CAD build for the part. Positions are in the model's coordinates, mm. A direction names the side the tool comes from. Give positions to 0.01 mm unless a question says otherwise; leave off trailing zeros. Loops run counter-clockwise (first coordinate to the right, second up) from the corner with the lowest first, then second, coordinate; pieces in that order, holes last. Notation, with made-up numbers: M -38.75,-17.75 L -17.75,-17.75 A35 cw -17.75,15.25 Z; hole C -26.5,54 d2. An arc over 180 degrees is marked long. Answer as CSV lines item,"result".
```python
from build123d import *

# Parameters (mm, degrees)
F2_R            = 1.27
F5_D            = 4.826
F5_DEPTH        = 7.62
F5_START        = 0.0546078
F5_TIP          = 1.4498766737
F5_COPIES_COUNT = 5


# Not quite as in the source:
# - a pattern or mirror of a feature is missing from the dataset's text; its kind, count and spacing are read off the source's solid


with BuildPart() as f1:
    # F0 (on Right) → F1 (revolve)
    with BuildSketch(Plane.YZ):
        Polygon((-6.35, 50.8), (6.35, 50.8), (6.35, 53.34), (-8.89, 53.34), (-8.89, 40.64), (-135.9245181084, 40.64), (-141.0045181084, 40.64), (-141.0045181084, 0), (-135.9245181084, 0), (-135.9245181084, 38.1), (-6.35, 38.1), align=None)
    revolve(axis=Axis((0, -59.97428298, 0), (0, -1, 0)))

    # F2
    f2_edges = [f1.edges().sort_by_distance(p)[0] for p in [
        (0, -6.35, -38.1),
        (0, -6.35, -50.8),
        (0, -8.89, -40.64),
        (0, -135.924518, -38.1),
    ]]
    fillet(f2_edges, radius=F2_R)

    # F5
    # its depths count from where the whole tool has entered the part; down to there all is cleared
    with Locations(Plane.XY.offset(53.34).offset(-F5_START)):
        with Locations((0, 0)):
            f5 = Hole(F5_D / 2, depth=F5_DEPTH)
            with Locations((0, 0, -(F5_DEPTH + F5_TIP / 2))):  # 118° drill point
                Cone(0, F5_D / 2, F5_TIP, mode=Mode.SUBTRACT)

    # F5_copies: F5 ×5 about axis
    f5_copies_axis = Axis((0, 0, 0), (0, 1, 0))
    for i in range(1, F5_COPIES_COUNT):
        add(f5.rotate(f5_copies_axis, i * 360 / F5_COPIES_COUNT), mode=Mode.SUBTRACT)


solid = f1.part
```
Q1. Pin check, flat tips, straight feed: P1, Ø5, axis at x = -32, y = -77.5, coming from the -Z side; P2, Ø4, axis at x = -9.5, y = -92.5, coming from the +Z side; P3, Ø3, axis at x = 34, y = -88.5, coming from the -Z side. Stop position of each tip, or through.
Solution:
P1,"stops at z = -27.95"
P2,"stops at z = 39.94"
P3,"stops at z = -24.4"
Q2. Cut at D-D (y = -68). Write the cut outline in (x, z), and give its area (3 significant figures).
Solution:
outline,"C 0,0 d81.28; hole C 0,0 d76.2"
area,"628 mm²"
Q3. Wall check: line 1 (X direction, y = -33.5, z = 1); line 2 (Z direction, x = 0, y = -43.5); line 3 (X direction, y = -2.25, z = 0). Give the ranges that are in metal, low to high. Write a range as [from, to].
Solution:
line 1,"x = [-40.63, -38.09], [38.09, 40.63]"
line 2,"z = [-40.64, -38.1], [38.1, 40.64]"
line 3,"x = [-53.34, -50.8], [50.8, 53.34]"
Q4. Cut at A-A (x = 0). Write the cut outline in (y, z), and give its area (3 significant figures).
Solution:
outline,"M -141,-40.64 L -10.16,-40.64 A1.27 cw -8.89,-41.91 L -8.89,-53.34 L 6.35,-53.34 L 6.35,-50.8 L -5.08,-50.8 A1.27 cw -6.35,-49.53 L -6.35,-39.37 A1.27 ccw -7.62,-38.1 L -134.65,-38.1 A1.27 cw -135.92,-36.83 L -135.92,36.83 A1.27 cw -134.65,38.1 L -7.62,38.1 A1.27 ccw -6.35,39.37 L -6.35,49.53 A1.27 cw -5.08,50.8 L -2.41,50.8 L -2.41,53.34 L -8.89,53.34 L -8.89,41.91 A1.27 cw -10.16,40.64 L -141,40.64 Z; M 2.41,50.8 L 6.35,50.8 L 6.35,53.34 L 2.41,53.34 Z"
area,"1,190 mm²"
Q5. Mould opens along Z. For faces 4 (the cylindrical face through (49.13, -2.14, 17.14)), 5 (the cylindrical face through (1.915, -1.468, 52.023)), 6 (the cylindrical face through (-40.294, -76.498, -5.291)), 7 (the cylindrical face through (23.183, -70.248, -30.235)) say: released by +Z, released by -Z, zero draft, split by the parting line, or undercut.
Solution:
face 4,"undercut"
face 5,"zero draft"
face 6,"split by the parting line"
face 7,"undercut"
Q6. Cut at B-B (z = 0). Write the cut outline in (x, y), and give its area (3 significant figures).
Solution:
outline,"M -53.34,-8.89 L -41.91,-8.89 A1.27 cw -40.64,-10.16 L -40.64,-141 L 40.64,-141 L 40.64,-10.16 A1.27 cw 41.91,-8.89 L 53.34,-8.89 L 53.34,6.35 L 50.8,6.35 L 50.8,-5.08 A1.27 cw 49.53,-6.35 L 39.37,-6.35 A1.27 ccw 38.1,-7.62 L 38.1,-134.65 A1.27 cw 36.83,-135.92 L -36.83,-135.92 A1.27 cw -38.1,-134.65 L -38.1,-7.62 A1.27 ccw -39.37,-6.35 L -49.53,-6.35 A1.27 cw -50.8,-5.08 L -50.8,6.35 L -53.34,6.35 Z"
area,"1,200 mm²"
Q7. Cut at C-C (y = 0). Write the cut outline in (x, z).
Solution:
outline,"M -51.42,14.17 A53.34 ccw -33.27,-41.69 L -31.78,-39.63 A50.8 cw -49,13.39 Z; M -49.93,18.76 L -47.51,17.98 A50.8 cw -2.41,50.74 L -2.41,53.29 A53.34 ccw Z; M -29.37,-44.53 A53.34 ccw 29.37,-44.53 L 27.87,-42.47 A50.8 cw -27.87,-42.47 Z; M 2.41,50.74 A50.8 cw 47.51,17.98 L 49.93,18.76 A53.34 ccw 2.41,53.29 Z; M 31.78,-39.63 L 33.27,-41.69 A53.34 ccw 51.42,14.17 L 49,13.39 A50.8 cw Z"
Q8. Which spindle directions (+Z, -Z, +X, -X, +Y, -Y) get a long thin tool onto all of the face, cutting with end or side? Do faces 1 (the flat face through (-1, -135.925, 1)), 2 (the flat face through (35.3, -8.89, 23.5)), 3 (the cylindrical face through (-50.188, 0.725, 13.887)). Say none if no direction does.
Solution:
face 1,"+Y"
face 2,"-Y"
face 3,"none"
